Verification items for the finished model (mm, model axes). Round coordinates to 2 decimals unless told otherwise and drop trailing zeros. Loops run counter-clockwise (first coordinate to the right, second up) from the corner with the lowest first, then second, coordinate; pieces in that order, holes last. Notation, with made-up numbers: (54, 21) -> (74, 21) arc R33 ccw to (74, 50) -> close; hole circle Ø9 at (13, -31). An arc over 180 degrees is marked (long way). Write item = value, one per line.
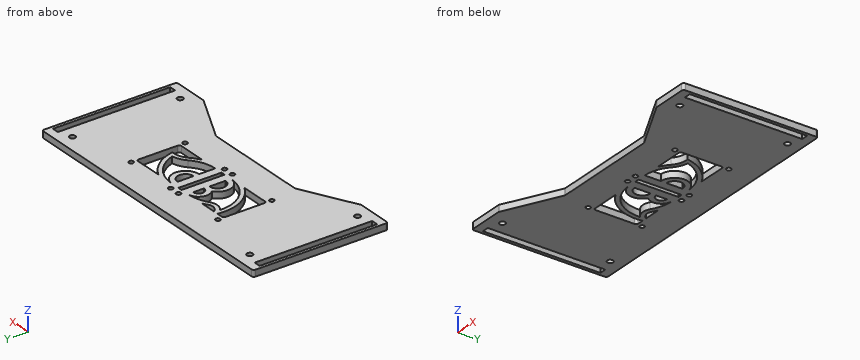
Autodesk Inventor part; units mm, degrees
ref_plane "YZ Plane" through (0, 0, 0) normal (1, 0, 0) x (0, 1, 0)
ref_plane "XZ Plane" through (0, 0, 0) normal (0, 1, 0) x (-1, 0, 0)
ref_plane "XY Plane" through (0, 0, 0) normal (0, 0, 1) x (1, 0, 0)
sketch "Sketch1" plane through (0, 0, 0) normal (0, 0, 1) x (1, 0, 0)
  line L0 (0, 0) -> (0, 125)
  line L1 (0, 125) -> (268, 125)
  line L2 (268, 125) -> (268, 0)
  line L3 (268, 0) -> (0, 0)
  point P0 (134, 125)
  dimension "d1" = 125
  dimension "d2" = 268
extrude "Extrusion1" add sketch "Sketch1" along normal blind 6
sketch "Sketch2" plane through (0, 0, 6) normal (0, 0, 1) x (1, 0, 0)
  line L0 (0, 0) -> (268, 0)
  line L1 (268, 0) -> (268, 125)
  line L2 (34, 0) -> (84, 25)
  line L3 (84, 25) -> (184, 25)
  line L4 (184, 25) -> (234, 0)
  line L5 (234, 0) -> (34, 0)
  line L6 (0, 125) -> (0, 0)
  dimension "d6" = 25
  dimension "d7" = 34
  dimension "d9" = 50
  dimension "d47" = 34
extrude "Extrusion2" cut sketch "Sketch2" against normal through all
sketch "Sketch7" plane through (0, 0, 6) normal (0, 0, 1) x (1, 0, 0)
  line L0 (268, 0) -> (268, 125)
  line L1 (268, 125) -> (0, 125)
  line L2 (0, 125) -> (0, 0)
  line L3 (0, 0) -> (34, 0)
  circle A0 centre (246.5, 12.5) radius 2.7
  circle A1 centre (246.5, 112.5) radius 2.7
  circle A2 centre (21.5, 12.5) radius 2.7
  circle A3 centre (21.5, 112.5) radius 2.7
  line L4 (2.875, 8.1) -> (9.125, 8.1)
  line L5 (9.125, 8.1) -> (9.125, 117)
  line L6 (9.125, 117) -> (2.875, 117)
  line L7 (2.875, 117) -> (2.875, 8.1)
  line L8 (2.875, 8.1) -> (9.125, 117) construction
  line L9 (9.125, 8.1) -> (2.875, 117) construction
  line L10 (258.875, 8.1) -> (265.125, 8.1)
  line L11 (265.125, 8.1) -> (265.125, 117)
  line L12 (265.125, 117) -> (258.875, 117)
  line L13 (258.875, 117) -> (258.875, 8.1)
  line L14 (258.875, 8.1) -> (265.125, 117) construction
  line L15 (265.125, 8.1) -> (258.875, 117) construction
  point P0 (6, 62.55)
  point P1 (262, 62.55)
  point P2 (6, 62.55)
  point P3 (262, 62.55)
  dimension "d48" = 21.5
  dimension "d49" = 21.5
  dimension "d50" = 12.5
  dimension "d51" = 12.5
  dimension "d56" = 2.875
  dimension "d57" = 6.25
  dimension "d58" = 2.875
  dimension "d60" = 8
  dimension "d61" = 5.4
  dimension "d62" = 108.9
  dimension "d66" = 8.1
extrude "Extrusion5" cut sketch "Sketch7" against normal through all
fillet "Fillet1" radius 2 8 edges at (268, 125, 3) (268, 0, 3) (234, 0, 3) (184, 25, 3) (84, 25, 3) (34, 0, 3) (0, 0, 3) (0, 125, 3)
sketch "Sketch8" plane through (0, 0, 6) normal (0, 0, 1) x (1, 0, 0)
  line L0 (9.125, 8.1) -> (2.875, 8.1)
  line L1 (84.4721, 25) -> (183.5279, 25)
  line L2 (266, 125) -> (2, 125)
  line L3 (79, 50) -> (129, 50) construction
  line L4 (129, 50) -> (129, 100) construction
  line L5 (129, 100) -> (79, 100) construction
  line L6 (79, 100) -> (79, 50) construction
  line L7 (79, 50) -> (129, 100) construction
  line L8 (129, 50) -> (79, 100) construction
  line L9 (139, 50) -> (189, 50) construction
  line L10 (189, 50) -> (189, 100) construction
  line L11 (189, 100) -> (139, 100) construction
  line L12 (139, 100) -> (139, 50) construction
  line L13 (139, 50) -> (189, 100) construction
  line L14 (189, 50) -> (139, 100) construction
  line L15 (104, 75) -> (164, 75) construction
  line L16 (134, 75) -> (134, 25) construction
  circle A0 centre (79, 100) radius 2.15
  circle A1 centre (129, 100) radius 2.15
  circle A2 centre (139, 100) radius 2.15
  circle A3 centre (189, 100) radius 2.15
  circle A4 centre (189, 50) radius 2.15
  circle A5 centre (139, 50) radius 2.15
  circle A6 centre (129, 50) radius 2.15
  circle A7 centre (79, 50) radius 2.15
  point P0 (0, 0)
  dimension "d67" = 50
  dimension "d68" = 60
  dimension "d69" = 100
  dimension "d70" = 25
  dimension "d71" = 4.3
extrude "Extrusion6" cut sketch "Sketch8" against normal blind 10
sketch "Sketch9" plane through (0, 0, 6) normal (0, 0, 1) x (1, 0, 0)
  circle A0 centre (79, 100) radius 2.15
  circle A1 centre (79, 50) radius 2.15
  line L0 (9.125, 117) -> (9.125, 8.1)
  line L1 (9.125, 8.1) -> (2.875, 8.1)
  line L2 (84.4721, 25) -> (183.5279, 25)
  line L3 (132, 55) -> (136, 55)
  line L4 (136, 55) -> (136, 95)
  line L5 (136, 95) -> (132, 95)
  line L6 (132, 95) -> (132, 55)
  line L7 (132, 55) -> (136, 95) construction
  line L8 (136, 55) -> (132, 95) construction
  line L9 (134, 25) -> (134, 75) construction
  line L10 (144, 90) -> (144, 75)
  arc A2 (144, 75) -> (144, 90) centre (144, 82.5) ccw
  arc A3 (144, 70) -> (144, 95) centre (144, 82.5) ccw
  line L11 (144, 70) -> (144, 55)
  arc A4 (178, 70) -> (144, 95) centre (144, 59.38) ccw
  arc A5 (178, 70) -> (166, 64) centre (181.2699, 48.4602) ccw
  arc A6 (144, 55) -> (166, 64) centre (144, 86.3889) ccw
  line L12 (144, 95) -> (136, 95) construction
  line L13 (136, 55) -> (144, 55) construction
  line L14 (161.3482, 95) -> (189, 95)
  line L15 (189, 95) -> (189, 55)
  line L16 (189, 55) -> (160.3435, 55)
  arc A7 (183.0358, 66.1589) -> (161.3482, 95) centre (144, 59.38) ccw
  arc A8 (160.3435, 55) -> (168.8035, 61.1469) centre (144, 86.3889) ccw
  arc A9 (183.0358, 66.1589) -> (168.8035, 61.1469) centre (181.2699, 48.4602) ccw
  line L17 (124, 75) -> (124, 60)
  line L18 (124, 90) -> (124, 80)
  arc A10 (124, 90) -> (124, 80) centre (124, 85) ccw
  arc A11 (124, 75) -> (124, 60) centre (124, 67.5) ccw
  arc A12 (117.0015, 77.8571) -> (124, 55) centre (124, 67.5) ccw
  arc A13 (124, 95) -> (117.0015, 77.8571) centre (124, 85) ccw
  line L19 (132, 95) -> (124, 95) construction
  line L20 (132, 55) -> (124, 55) construction
  arc A14 (124, 95) -> (104, 89) centre (124, 58.6667) ccw
  arc A15 (90, 90) -> (104, 89) centre (97.652, 98.6278) ccw
  arc A16 (90, 90) -> (124, 55) centre (124, 89.0143) ccw
  line L21 (86.4599, 95) -> (79, 95)
  line L22 (79, 95) -> (79, 55)
  line L23 (79, 55) -> (107.0261, 55)
  arc A17 (86.4599, 95) -> (107.0261, 55) centre (124, 89.0143) ccw
  arc A18 (91.051, 95) -> (101.7982, 92.3394) centre (97.652, 98.6278) ccw
  arc A19 (106.4881, 95) -> (101.7982, 92.3394) centre (124, 58.6667) ccw
  line L24 (91.051, 95) -> (106.4881, 95)
  point P0 (0, 0)
  point P1 (140, 55)
  dimension "d74" = 4
  dimension "d75" = 40
  dimension "d76" = 50
  dimension "d77" = 25
  dimension "d78" = 12.5
  dimension "d79" = 5
  dimension "d80" = 8
  dimension "d81" = 22
  dimension "d82" = 15
  dimension "d83" = 34
  dimension "d84" = 9
  dimension "d85" = 4
  dimension "d86" = 4
  dimension "d87" = 55
  dimension "d88" = 8
  dimension "d89" = 5
  dimension "d90" = 10
  dimension "d91" = 5
  dimension "d92" = 34
  dimension "d93" = 35
  dimension "d94" = 20
  dimension "d95" = 6
  dimension "d96" = 55
  dimension "d97" = 4
  dimension "d99" = 4
extrude "Extrusion7" cut sketch "Sketch9" against normal blind 10 contours L6 L5 L4 L3 | A2 L10 | A3 A4 A5 A6 L11 | L14 L15 L16 A8 A9 A7 | L17 A11 | L18 A10 | A12 A16 A15 A14 A13 | A17 L23 L22 L21 | L24 A19 A18
fillet "Fillet2" radius 2 4 edges at (79, 95, 3) (79, 55, 3) (189, 55, 3) (189, 95, 3)
equation "\"d7\" = d47"
equation "\"d49\" = d48"
equation "\"d51\" = d50"
equation "\"d58\" = d56"
equation "\"d70\" = -0.5 * d67 + 0.5 * d69"
equation "\"d77\" = 0.5 * d76"
equation "\"d86\" = d85"
equation "\"d89\" = d79"
equation "\"d91\" = d79"
equation "\"d97\" = d85"
properties part number "FrontPanel"
(1) Sectioned sample at D-D, the plane x = 198.5. Record the cut outline in (y, z).
Filled sheet:
outline = (17.75, 0) -> (125, 0) -> (125, 6) -> (17.75, 6) -> close
(2) Sectioned sample at C-C, the plane x = 246.5. Record the cut outline in (y, z), and give its area (3 significant figures).
Filled sheet:
outline = (0, 0) -> (9.8, 0) -> (9.8, 6) -> (0, 6) -> close; (15.2, 0) -> (109.8, 0) -> (109.8, 6) -> (15.2, 6) -> close; (115.2, 0) -> (125, 0) -> (125, 6) -> (115.2, 6) -> close
area = 685 mm2
(3) Go/stop test with flat-tipped pins: pin 1 Ø5 at (x, y) = (21.5, 12.5) entering from -Z; pin 2 Ø3 at (x, z) = (177.5, 1.5) entering from -Y. Record where each tip stops, or that it passes through.
Filled sheet:
pin_1 = through
pin_2 = 25
(4) Sectioned sample at B-B, the plane y = 21. Record the cut outline in (x, z) (3 decimals), and give its area (3 significant figures).
Filled sheet:
outline = (0, 0) -> (2.875, 0) -> (2.875, 6) -> (0, 6) -> close; (9.125, 0) -> (76, 0) -> (76, 6) -> (9.125, 6) -> close; (192, 0) -> (258.875, 0) -> (258.875, 6) -> (192, 6) -> close; (265.125, 0) -> (268, 0) -> (268, 6) -> (265.125, 6) -> close
area = 837 mm2
(5) Sectioned sample at A-A, the plane y = 112.5. Record the cut outline in (x, z) (3 decimals), and give its area (3 significant figures).
Filled sheet:
outline = (0, 0) -> (2.875, 0) -> (2.875, 6) -> (0, 6) -> close; (9.125, 0) -> (18.8, 0) -> (18.8, 6) -> (9.125, 6) -> close; (24.2, 0) -> (243.8, 0) -> (243.8, 6) -> (24.2, 6) -> close; (249.2, 0) -> (258.875, 0) -> (258.875, 6) -> (249.2, 6) -> close; (265.125, 0) -> (268, 0) -> (268, 6) -> (265.125, 6) -> close
area = 1,470 mm2
(6) Material ranges on probe 1 along X at (y, z) = (109, 5.2) (3 decimals); probe 2 along X at (y, z) = (113, 3.75) (3 decimals); probe 3 along Y at (x, z) = (129, 3.3), recorded low to high. Write a range as from..to.
Filled sheet:
probe_1 = 0..2.875, 9.125..258.875, 265.125..268
probe_2 = 0..2.875, 9.125..18.847, 24.153..243.847, 249.153..258.875, 265.125..268
probe_3 = 25..47.85, 52.15..97.85, 102.15..125
